CAD build for the part. Positions are in the model's coordinates, mm. Coordinates: 2 decimals unless noted, no trailing zeros. Loops run counter-clockwise (first coordinate to the right, second up) from the corner with the lowest first, then second, coordinate; pieces in that order, holes last.
1) Saw through at A-A, the plane y = 1. Write the cut outline in (x, z).
2) Saw through at C-C, the plane x = 34.5. Write the cut outline in (y, z).
3) Pin check, flat tips, straight feed: pin 1 Ø10 at (x, z) = (38.5, -9) entering from -Y; pin 2 Ø1 at (y, z) = (-13.5, -9) entering from +X; pin 3 Ø6 at (x, y) = (18.5, 13.5) entering from +Z. Stop position of each tip, or through.
4) Saw through at B-B, the plane z = -13. Write the cut outline in (x, y), and give its area (3 significant figures).
5) Wall check: line 1 along Z through (x, y) = (54.5, 4); line 2 along Z through (x, y) = (25, 2); line 3 along X through (y, z) = (18.5, -15). Give the ranges that are in metal, low to high.
Autodesk Inventor part; units mm, degrees
ref_plane "工作平面1" through (10, 22, 0) normal (-0.4554, -0.6295, -0.6295) x (0.8102, 0, -0.5861)
ref_plane "YZ Plane" through (0, 0, 0) normal (1, 0, 0) x (0, 1, 0)
ref_plane "XZ Plane" through (0, 0, 0) normal (0, 1, 0) x (-1, 0, 0)
sketch "草圖1" plane through (0, 0, 0) normal (0, 1, 0) x (-1, 0, 0)
  line L0 (0, 0) -> (-57, 0)
  line L1 (-57, 0) -> (-57, -44)
  line L2 (-57, -44) -> (0, -44)
  line L3 (0, -44) -> (0, 0)
  dimension "d0" = 57
  dimension "d1" = 44
extrude "擠出1" add sketch "草圖1" along normal mid plane 44
sketch "草圖2" plane through (0, 22, 0) normal (0, 1, 0) x (1, 0, 0)
  line L0 (0, 0) -> (57, 0)
  line L1 (10, 0) -> (57, 14)
  line L2 (57, 0) -> (57, 44)
  dimension "d4" = 10
  dimension "d5" = 30
extrude "擠出2" cut sketch "草圖2" against normal blind 60
sketch "草圖3" plane through (57, -22, -44) normal (1, 0, 0) x (0, 0, -1)
  line L0 (-30, 24) -> (-10, 44)
  line L1 (0, 44) -> (-44, 44)
  line L2 (-30, 44) -> (-30, 0)
  point P0 (-44, 22)
  point P1 (-30, 2)
  dimension "d8" = 20
  dimension "d9" = 20
ref_plane "工作平面1" through (10, 22, 0) normal (-0.4554, -0.6295, -0.6295) x (0.8102, 0, -0.5861)
sketch "草圖4" plane through (10, 22, 0) normal (-0.4554, -0.6295, -0.6295) x (0.8102, 0, -0.5861)
  line L0 (-15.1543, -12.3218) -> (93.717, -12.3218)
  line L1 (93.717, -12.3218) -> (93.717, 28.8166)
  line L2 (93.717, 28.8166) -> (-15.1543, 28.8166)
  line L3 (-15.1543, 28.8166) -> (-15.1543, -12.3218)
  point P0 (-8.1022, 13.4037)
extrude "擠出3" cut sketch "草圖4" against normal blind 40
mirror "鏡射1" about plane through (0, 0, 0) normal (0, 1, 0) of "擠出3"
properties part number "62"
Data:
1. outline: (0, -44) - (57, -44) - (57, -14) - (10, 0) - (0, 0) - close
2. outline: (-22, -44) - (22, -44) - (22, -17.73) - (11.57, -7.3) - (-11.57, -7.3) - (-22, -17.73) - close
3. pin 1: stops at y = -16.55
3. pin 2: stops at x = 35.16
3. pin 3: stops at z = -1.64
4. outline: (0, -22) - (27.97, -22) - (53.64, -3.42) - (53.64, 3.42) - (27.97, 22) - (0, 22) - close
4. area: 1,880 mm2
5. line 1: z = -44 to -14.2
5. line 2: z = -44 to -4.47
5. line 3: x = 0 to 35.57
